```python
from build123d import *

# Parameters (mm, degrees)
CUT_EXTRUDE1_DEPTH      = 39.29792341
CUT_EXTRUDE1_DEPTH_BACK = 39.29792341
CUT_EXTRUDE2_DEPTH      = 39.297923559
CUT_EXTRUDE2_DEPTH_BACK = 39.297923559
CUT_EXTRUDE3_DEPTH      = 20
CUT_EXTRUDE3_DEPTH_BACK = 10
SKETCH5_R               = 1.49
SKETCH6_R               = 9.525
BOSS_EXTRUDE1_DEPTH     = 4.32
SKETCH7_W               = 30.231147159
SKETCH7_H               = 26.898579755
CUT_EXTRUDE4_DEPTH      = 5.43


with BuildPart() as part:
    # Sketch1 → Revolve1 (revolve)
    with BuildSketch(Plane(origin=(0, 0, 0), x_dir=(0, 0, -1), z_dir=(1, 0, 0))):
        Polygon((-34.925, 11.1125), (-34.925, 9.525), (-15.925, 9.525), (-15.925, 0), (11.1125, 0), (11.1125, 11.1125), align=None)
    revolve(axis=Axis((0, 0, 0), (0, 0, 1)))

    # Sketch3 → Cut-Extrude1 (cut, two sides: drawn at the far end of the back side and taken through both)
    with BuildSketch(Plane(origin=(0, 0, 0), x_dir=(0, 0, -1), z_dir=(1, 0, 0)).offset(-CUT_EXTRUDE1_DEPTH_BACK)):
        with BuildLine():
            Line((11.1125, 11.1125), (-10.233333333, 11.1125))
            Line((-10.233333333, 11.1125), (-10.233333333, 8.466666667))
            ThreePointArc((-10.233333333, 8.466666667), (-8.993418707, 5.47324796), (-6, 4.233333333))
            Line((-6, 4.233333333), (0, 4.233333333))
            ThreePointArc((0, 4.233333333), (4.233333333, 0), (0, -4.233333333))
            Line((0, -4.233333333), (-6, -4.233333333))
            ThreePointArc((-6, -4.233333333), (-8.993418707, -5.47324796), (-10.233333333, -8.466666667))
            Line((-10.233333333, -8.466666667), (-10.233333333, -11.1125))
            Line((-10.233333333, -11.1125), (11.1125, -11.1125))
            Line((11.1125, -11.1125), (11.1125, 11.1125))
        make_face()
    extrude(amount=CUT_EXTRUDE1_DEPTH + CUT_EXTRUDE1_DEPTH_BACK, mode=Mode.SUBTRACT)

    # Sketch4 → Cut-Extrude2 (cut, two sides: drawn at the far end of the back side and taken through both)
    with BuildSketch(Plane(origin=(0, 0, 0), x_dir=(1, 0, 0), z_dir=(0, 1, 0)).offset(-CUT_EXTRUDE2_DEPTH_BACK)):
        with BuildLine():
            Line((-2.825, -10.233333333), (2.825, -10.233333333))
            ThreePointArc((2.825, -10.233333333), (5.07006403, -9.303397364), (6, -7.058333333))
            Line((6, -7.058333333), (6, 4.233333333))
            Line((6, 4.233333333), (-6, 4.233333333))
            Line((-6, 4.233333333), (-6, -7.058333333))
            ThreePointArc((-6, -7.058333333), (-5.07006403, -9.303397364), (-2.825, -10.233333333))
        make_face()
    extrude(amount=CUT_EXTRUDE2_DEPTH + CUT_EXTRUDE2_DEPTH_BACK, mode=Mode.SUBTRACT)

    # Sketch5 → Cut-Extrude3 (cut, two sides: drawn at the far end of the back side and taken through both)
    with BuildSketch(Plane(origin=(-6, 0, 0), x_dir=(0, 0, -1), z_dir=(1, 0, 0)).offset(-CUT_EXTRUDE3_DEPTH_BACK)):
        with Locations(Location((0, 0, 0), (0, 0, 180))):
            Circle(SKETCH5_R)
    extrude(amount=CUT_EXTRUDE3_DEPTH + CUT_EXTRUDE3_DEPTH_BACK, mode=Mode.SUBTRACT)

    # Sketch6 → Boss-Extrude1 (add)
    with BuildSketch(Plane.XY.offset(15.925)):
        with Locations(Location((0, 0, 0), (0, 0, 90))):
            Circle(SKETCH6_R)
    extrude(amount=BOSS_EXTRUDE1_DEPTH)

    # Sketch7 → Cut-Extrude4 (cut)
    with BuildSketch(Plane.XY.offset(34.925)):
        with Locations((1.508431665, -0.773631718)):
            Rectangle(SKETCH7_W, SKETCH7_H)
    extrude(amount=-CUT_EXTRUDE4_DEPTH, mode=Mode.SUBTRACT)


solid = part.part
```
The listing builds one solid part. Answer for the finished solid, in the listing's coordinates (mm). A direction names the side the tool comes from. Coordinates: 2 decimals unless noted, no trailing zeros. Loops run counter-clockwise (first coordinate to the right, second up) from the corner with the lowest first, then second, coordinate; pieces in that order, holes last. Notation, with made-up numbers: (12, 5.25) -> (47, 5.25) arc R21 cw to (47, 24.25) -> close; hole circle Ø5 at (55, 67). An arc over 180 degrees is marked (long way). Use one line per item in the form item = value. Start each with the question number.
Item 1: The part is cut by section B-B on z = 8. Determine the outline of the cut face in (x, y) (1 decimal), then the cut area to 3 significant figures.
Item 2: The part is cut by section A-A on y = 0. Count the separate pieces of the cut face and the enclosed holes in it, then the cut area to 3 significant figures.
Item 3: A tool of negligible diameter and unlimited length cuts with its end or side. For faces 3 (the face through (6, 0, 3)), 4 (the face through (0, 0, 20.245)), 5 (the face through (-8, 4.233, 3)), 6 (the face through (8, -4.233, 3)), from which of +Z, -Z, +X, -X, +Y, -Y can it reach the whole face along a straight path? Write none if from no direction.
Item 4: The part is cut by section D-D on x = -7.75. Determine the outline of the cut face in (y, z) (3 decimals), then the cut area to 3 significant figures.
Item 5: Consider L1, parallel to X at y = 0, z = 25 (1 decimal); L2, parallel to Y at x = -9.5, z = 0; L3, parallel to X at y = 0.5, z = 7.5. Determine where each line is inside the solid, lowest interval first. Write a range as [from, to].
Item 6: The part is cut by section C-C on x = 0. Determine the outline of the cut face in (y, z) (1 decimal).
Item 7: Flat-ended cylindrical pins translate along their axes: pin 1 Ø2 at (x, z) = (8, 4) entering from +Y; pin 2 Ø3 at (x, y) = (3.5, 3) entering from +Z (3 decimals); pin 3 Ø4.5 at (x, z) = (7.5, 2) entering from -Y; pin 4 Ø1.8 at (y, z) = (0, 0) entering from -X (1 decimal). Find the tip coordinate at first contact, or state that the pin passes through.
Item 8: The mould has two halves that part along X. Classify faces 1 (the face through (8, 4.233, 3)), 2 (the face through (0, 0, 10.233)): released by +X, released by -X, zero draft, split by the parting line, or undercut.
Answer key:
q1.outline = (-10.1, -4.7) -> (-5.9, -4.7) -> (-5.9, 4.7) -> (-10.1, 4.7) arc R11.1 ccw to start; (5.9, -4.7) -> (10.1, -4.7) arc R11.1 ccw to (10.1, 4.7) -> (5.9, 4.7) -> close
q1.area = 93.0 mm2
q2.separate_pieces = 3
q2.enclosed_holes = 0
q2.area = 374 mm2
q3.face_3 = -Z, +Y, -Y
q3.face_4 = +Z
q3.face_5 = -Z, +X, -X, +Y
q3.face_6 = -Z, +X, -X, -Y
q4.outline = (-7.964, 10.203) arc R4.233 cw to (-4.233, 6) -> (-4.233, 0) arc R4.233 ccw to (4.233, 0) -> (4.233, 6) arc R4.233 cw to (7.964, 10.203) -> (7.964, 29.495) -> (5.537, 29.495) -> (5.537, 20.245) -> (-5.537, 20.245) -> (-5.537, 29.495) -> (-7.964, 29.495) -> close; hole circle Ø2.98 at (0, 0)
q4.area = 320 mm2
q5.L1 = [-11.1, -9.5], [9.5, 11.1]
q5.L2 = [-4.23, -1.49], [1.49, 4.23]
q5.L3 = [-11.1, -5.97], [5.97, 11.1]
q6.outline = (-11.1, 10.2) -> (11.1, 10.2) -> (11.1, 29.5) -> (9.5, 29.5) -> (9.5, 20.2) -> (-9.5, 20.2) -> (-9.5, 29.5) -> (-11.1, 29.5) -> close
q7.pin_1 = 4.23
q7.pin_2 = 20.245
q7.pin_3 = -4.23
q7.pin_4 = through
q8.face_1 = zero draft
q8.face_2 = undercut
